Input: dimensioned drawing with shaded views. Units: mm. Origin: part minimum x, y, z. Round coordinates to 2 decimals unless told otherwise and drop trailing zeros. Loops run counter-clockwise (first coordinate to the right, second up) from the corner with the lowest first, then second, coordinate; pieces in that order, holes last. Notation, with made-up numbers: (-17.75, 69.5) - (30.25, 69.5) arc R17 cw to (30.25, 96.5) - close; hole circle Ø10 at (-13.5, -23.5). An arc over 180 degrees is marked (long way). Answer as a JSON object with one key per item and string values. Group by question number.
Item 1: Section D-D (x = 25.25). Return the cut outline in (y, z) (1 decimal), plus the area to 3 significant figures.
Item 2: First-contact query: pin 1 (1.5 mm diameter, centred on x = 10, y = 25.5, fed in from -Z) (1 decimal); pin 2 (10 mm diameter, centred on x = 10.5, z = 55, fed in from +Y); pin 3 (12 mm diameter, centred on x = 13.5, z = 19.5, fed in from +Y) (1 decimal). Flat tips, straight axial feed; report the tip coordinate or a pass-through.
Item 3: Section B-B (x = 18.5). Return the cut outline in (y, z) (1 decimal), plus the area to 3 significant figures.
Item 4: Section A-A (y = 17). Return the cut outline in (x, z).
Item 5: Section C-C (z = 15.5). Return the cut outline in (x, y) (1 decimal), plus the area to 3 significant figures.
Item 6: Draft query along Y for the marked faces 1, 2 and 3. Return one class per face: released by +Y, released by -Y, zero draft, split by the parting line, or undercut.
Item 7: Line query: line 1 (X direction, y = 14, z = 83.5) (1 decimal); line 2 (Z direction, x = 8.75, y = 24); line 3 (X direction, y = 15, z = 76). Output: solid intervals per line, ascending.
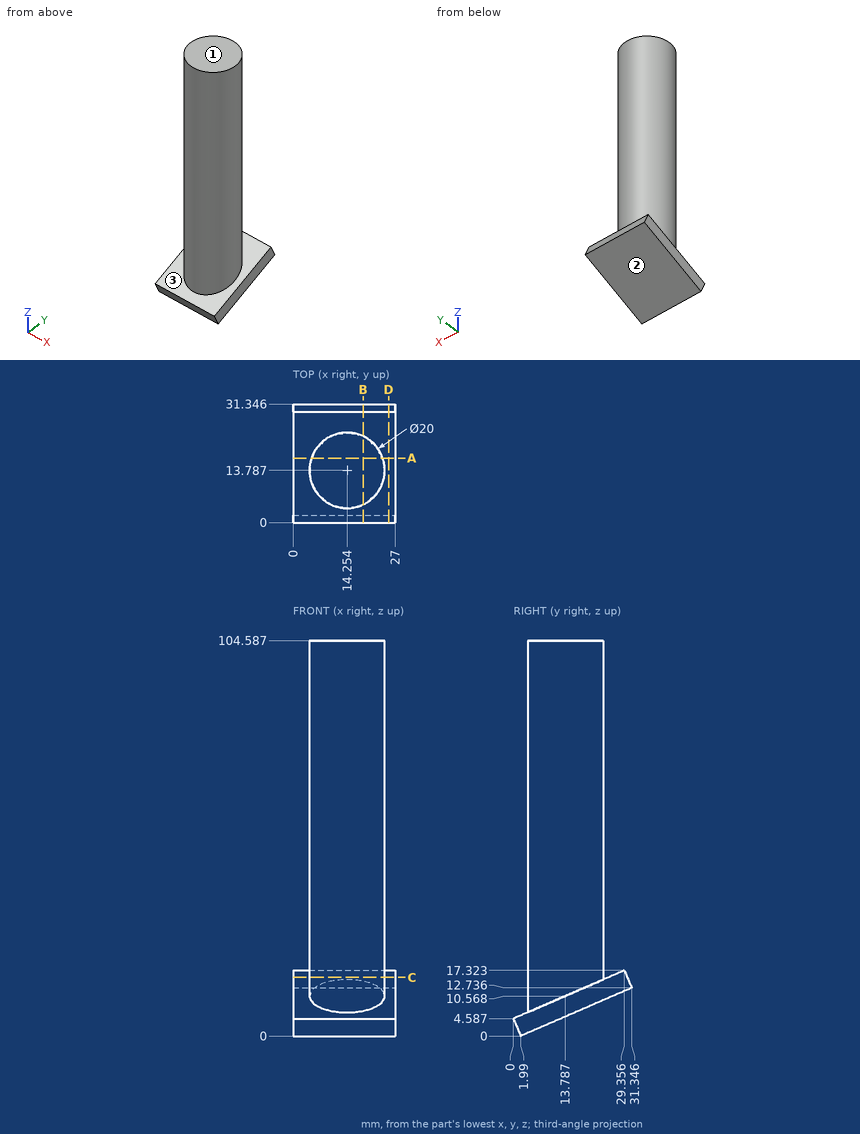
Values:
{
 "1": {"outline": "(0, 4.6) - (2, 0) - (31.3, 12.7) - (29.4, 17.3) - close", "area": "160 mm^2"},
 "2": {"pin 1": "stops at z = 9.9", "pin 2": "stops at y = 23.79", "pin 3": "stops at y = 31"},
 "3": {"outline": "(0, 4.6) - (2, 0) - (31.3, 12.7) - (29.4, 17.3) - (22.8, 14.5) - (22.8, 104.6) - (4.7, 104.6) - (4.7, 6.6) - close", "area": "1,860 mm^2"},
 "4": {"outline": "(0, 6.51) - (27, 6.51) - (27, 11.96) - (23.72, 11.96) - (23.72, 104.59) - (4.78, 104.59) - (4.78, 11.96) - (0, 11.96) - close"},
 "5": {"outline": "(0, 25.2) - (27, 25.2) - (27, 30.1) - (0, 30.1) - close; circle Ø20 at (14.3, 13.8)", "area": "449 mm^2"},
 "6": {"face 1": "zero draft", "face 2": "released by +Y", "face 3": "undercut"},
 "7": {"line 1": "x = 4.3 to 24.3", "line 2": "z = 9.55 to 15", "line 3": "x = 4.33 to 24.18"}
}
